from build123d import *

# Parameters (mm, degrees)
SKETCH2_R           = 11
BOSS_EXTRUDE1_DEPTH = 10
SKETCH4_R           = 19
SKETCH4_R_2         = 15
BOSS_EXTRUDE2_DEPTH = 10


with BuildPart() as part:
    # Sketch2 → Boss-Extrude1 (new body)
    with BuildSketch(Plane.XY):
        with BuildLine():
            Line((26.747478069, -30.009538766), (50.730734825, -63.019659758))
            ThreePointArc((50.730734825, -63.019659758), (60.147924382, -54.104640877), (68.019750294, -43.79952673))
            ThreePointArc((68.019750294, -43.79952673), (66.573956141, -21.631189606), (80.773849811, -4.546444618))
            ThreePointArc((80.773849811, -4.546444618), (80.462602989, 8.417511037), (78.084053221, 21.165197956))
            Line((78.084053221, 21.165197956), (39.278328629, 8.55645371))
            ThreePointArc((39.278328629, 8.55645371), (34.238034587, 11.124611797), (36.806192674, 16.16490584))
            Line((36.806192674, 16.16490584), (75.611917266, 28.773650086))
            ThreePointArc((75.611917266, 28.773650086), (70.043302078, 40.484821919), (62.675084101, 51.155828649))
            ThreePointArc((62.675084101, 51.155828649), (41.14496766, 56.631189606), (29.284418072, 75.415567558))
            ThreePointArc((29.284418072, 75.415567558), (16.858783013, 79.125636852), (4, 80.802753492))
            Line((4, 80.802753492), (4, 40))
            ThreePointArc((4, 40), (0, 36), (-4, 40))
            Line((-4, 40), (-4, 80.802753492))
            ThreePointArc((-4, 80.802753492), (-16.858783013, 79.125636852), (-29.284418072, 75.415567558))
            ThreePointArc((-29.284418072, 75.415567558), (-41.14496766, 56.631189606), (-62.675084101, 51.155828649))
            ThreePointArc((-62.675084101, 51.155828649), (-70.043302078, 40.484821919), (-75.611917266, 28.773650086))
            Line((-75.611917266, 28.773650086), (-36.806192674, 16.16490584))
            ThreePointArc((-36.806192674, 16.16490584), (-34.238034587, 11.124611797), (-39.278328629, 8.55645371))
            Line((-39.278328629, 8.55645371), (-78.084053221, 21.165197956))
            ThreePointArc((-78.084053221, 21.165197956), (-80.462602989, 8.417511037), (-80.773849811, -4.546444618))
            ThreePointArc((-80.773849811, -4.546444618), (-66.573956141, -21.631189606), (-68.019750294, -43.79952673))
            ThreePointArc((-68.019750294, -43.79952673), (-60.147924382, -54.104640877), (-50.730734825, -63.019659758))
            Line((-50.730734825, -63.019659758), (-26.747478069, -30.009538766))
            ThreePointArc((-26.747478069, -30.009538766), (-21.160269083, -29.124611797), (-20.275342114, -34.711820784))
            Line((-20.275342114, -34.711820784), (-44.25859887, -67.721941776))
            ThreePointArc((-44.25859887, -67.721941776), (-32.869840458, -73.92332893), (-20.636566513, -78.225424859))
            ThreePointArc((-20.636566513, -78.225424859), (0, -70), (20.636566513, -78.225424859))
            ThreePointArc((20.636566513, -78.225424859), (32.869840458, -73.92332893), (44.25859887, -67.721941776))
            Line((44.25859887, -67.721941776), (20.275342114, -34.711820784))
            ThreePointArc((20.275342114, -34.711820784), (21.160269083, -29.124611797), (26.747478069, -30.009538766))
        make_face()
        Circle(SKETCH2_R, mode=Mode.SUBTRACT)
    extrude(amount=BOSS_EXTRUDE1_DEPTH)

    # Sketch4 → Boss-Extrude2 (add)
    with BuildSketch(Plane(origin=(0, 0, 0), x_dir=(-1, 0, 0), z_dir=(0, 0, -1))):
        with Locations(Location((0, 0, 0), (0, 0, 180))):
            Circle(SKETCH4_R)
        Circle(SKETCH4_R_2, mode=Mode.SUBTRACT)
    extrude(amount=BOSS_EXTRUDE2_DEPTH)


solid = part.part
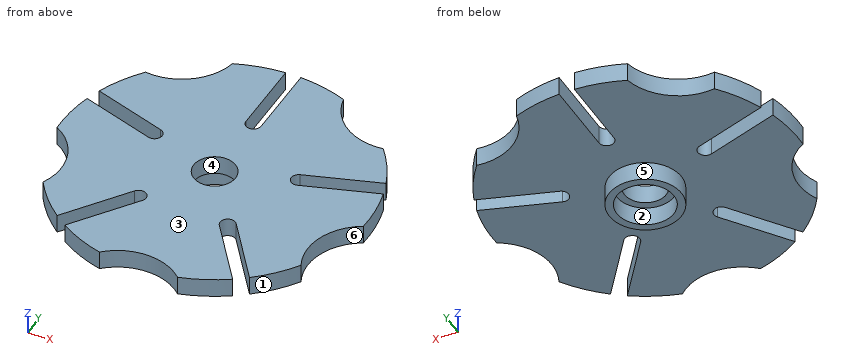
Read the model definition and answer for the solid it produces. Units are mm, in the model's axes. Face numbers are marked on the shaded views. A direction names the side the tool comes from. Round coordinates to 2 decimals unless told otherwise and drop trailing zeros. Order: outer loops, then holes, each group sorted by start corner. A loop starts at its lowest first (then second) coordinate and runs counter-clockwise, first axis right, second up.
1) The part is cut by section A-A on y = 0. Write down the section's boundary in (x, z).
2) For the marked faces 5 and 6, determine the directions among +Z, -Z, +X, -X, +Y, -Y from which every point of the face is accessible in a straight line to the end or side of a thin tool.
3) Flat-ended cylindrical pins translate along their axes: pin 1 (3 mm diameter, centred on x = 27.5, z = 5.5, fed in from -Y); pin 2 (3 mm diameter, centred on x = 20, y = 46.5, fed in from -Z); pin 3 (6 mm diameter, centred on y = -5, z = 2, fed in from +X). Find the tip coordinate at first contact, or state that the pin passes through.
4) The part is cut by section B-B on x = 0. Write down the section's boundary in (y, z), plus the area to 3 significant figures.
5) Straight lines are drawn through the part: L1, parallel to Y at x = 0, z = -7.25; L2, parallel to Y at x = 0, z = 5; L3, parallel to Y at x = 37.5, z = 1.5. For each, find the intervals that lie inside material, in ascending order.
6) The mould has two halves that part along Y. Classify the marked faces 1, 2, 3 and 4: released by +Y, released by -Y, zero draft, split by the parting line, or undercut.
7) The part is cut by section D-D on y = 38. Write down the section's boundary in (x, z).
Resolved:
1. outline: (-80.9, 0) - (-19, 0) - (-19, -10) - (-15, -10) - (-15, 0) - (-11, 0) - (-11, 10) - (-80.9, 10) - close; (11, 0) - (15, 0) - (15, -10) - (19, -10) - (19, 0) - (80.9, 0) - (80.9, 10) - (11, 10) - close
2. face 5: -Z
2. face 6: +Z, -Z, +X
3. pin 1: stops at y = -76.61
3. pin 2: stops at z = 0
3. pin 3: stops at x = 80.88
4. outline: (-70, 0) - (-19, 0) - (-19, -10) - (-15, -10) - (-15, 0) - (-11, 0) - (-11, 10) - (-70, 10) - close; (11, 0) - (15, 0) - (15, -10) - (19, -10) - (19, 0) - (36, 0) - (36, 10) - (11, 10) - close
4. area: 920 mm2
5. L1: y = -19 to -15, 15 to 19
5. L2: y = -70 to -11, 11 to 36
5. L3: y = -71.69 to -58.42, -44.81 to 8.4, 16.39 to 59.75
6. face 1: released by -Y
6. face 2: undercut
6. face 3: zero draft
6. face 4: undercut
7. outline: (-71.42, 0) - (-3.46, 0) - (-3.46, 10) - (-71.42, 10) - close; (3.46, 0) - (71.42, 0) - (71.42, 10) - (3.46, 10) - close
